```python
from build123d import *

# Parameters (mm, degrees)
F0_W     = 60
F0_H     = 40
F1_DEPTH = 10
F3_START = -20
F3_DEPTH = 20
F4_R     = 10
F5_DEPTH = 25


with BuildPart() as f1:
    # F0 (on Top) → F1 (new body)
    with BuildSketch(Plane.XY):
        with Locations((30, 20)):
            Rectangle(F0_W, F0_H)
    extrude(amount=F1_DEPTH)

    # F2 (on Front) → F3 (join)
    with BuildSketch(Plane.XZ.offset(F3_START)):
        with BuildLine():
            Line((50, 20), (40, 20))
            ThreePointArc((40, 20), (20, 40), (0, 20))
            Line((0, 20), (0, 10))
            Line((0, 10), (60, 10))
            ThreePointArc((60, 10), (57.0710678119, 17.0710678119), (50, 20))
        make_face()
    extrude(amount=-F3_DEPTH)

    # F4 (on face) → F5 (cut)
    with BuildSketch(Plane.XZ.offset(-20)):
        with Locations((20, 20)):
            Circle(F4_R)
    extrude(amount=-F5_DEPTH, mode=Mode.SUBTRACT)


solid = f1.part
```
Geometry check sheet. Reference: the model listing, model coordinates, mm. A direction names the side the tool comes from. Coordinates: 2 decimals unless noted, no trailing zeros. Order: outer loops, then holes, each group sorted by start corner. A loop starts at its lowest first (then second) coordinate and runs counter-clockwise, first axis right, second up. Notation, with made-up numbers: M 77,19.5 L 114,19.5 A18 cw 114,36.5 Z; hole C -18.75,7 d11. An arc over 180 degrees is marked long. One line per question, with ' | ' between items. Start each with the question number.
Item 1: Set-up check for faces 1 (the flat face through (30, 10, 10)), 2 (the cylindrical face through (57.15, 29.86, 16.99)): record each of +Z, -Z, +X, -X, +Y, -Y from which the full face is reachable in a straight line by a thin tool's end or side.
Item 2: Cross-section at B-B on z = 24.5. Enter the section's corners in (x, y), then the cut area to 3 significant figures.
Item 3: Cross-section at C-C on x = 41. Enter the section's corners in (y, z), then the cut area to 3 significant figures.
Item 4: Material ranges on L1, parallel to Z at x = 20, y = 32.25; L2, parallel to Y at x = 29, z = 32; L3, parallel to Z at x = 37.5, y = 12, recorded low to high. Write a range as [from, to].
Item 5: Gauge pin test, flat ends, axial feed: pin 1 (9 mm diameter, centred on x = 40.5, z = 23.5, fed in from -Y); pin 2 (22 mm diameter, centred on x = 36.5, y = 6, fed in from +Z); pin 3 (2 mm diameter, centred on y = 28.5, z = 28, fed in from +X) (3 decimals). Record the tip position at first contact, or that the pin passes through.
Item 6: Draft check along Z on faces 3 (the flat face through (30, 40, 16)), 4 (the cylindrical face through (29.54, 29.86, 23)), 5 (the flat face through (45, 30, 20)), 6 (the flat face through (30, 20, 0)). Enter one of: pulls with the +Z half, pulls with the -Z half, needs draft (parallel to the pull), parting line crosses it, or undercut.
Item 7: Cross-section at A-A on y = 23. Enter the section's corners in (x, z), then the cut area to 3 significant figures.
Item 8: Cross-section at D-D on x = 15. Enter the section's corners in (y, z), then the cut area to 3 significant figures.
Findings:
1) face 1: +Z, +X, -X, -Y | face 2: +Z, +X, +Y, -Y
2) outline: M 0.51,20 L 11.07,20 L 11.07,40 L 0.51,40 Z; M 28.93,20 L 39.49,20 L 39.49,40 L 28.93,40 Z | area: 422 mm²
3) outline: M 0,0 L 40,0 L 40,20 L 20,20 L 20,10 L 0,10 Z | area: 600 mm²
4) L1: z = [0, 10], [30, 40] | L2: y = [20, 40] | L3: z = [0, 10]
5) pin 1: stops at y = 20 | pin 2: stops at z = 10 | pin 3: stops at x = 38.735
6) face 3: needs draft | face 4: undercut | face 5: pulls with the +Z half | face 6: pulls with the -Z half
7) outline: M 0,0 L 60,0 L 60,10 A10 ccw 50,20 L 40,20 A20 ccw 0,20 Z; hole C 20,20 d20 | area: 1,490 mm²
8) outline: M 0,0 L 40,0 L 40,11.34 L 20,11.34 L 20,10 L 0,10 Z; M 20,28.66 L 40,28.66 L 40,39.36 L 20,39.36 Z | area: 641 mm²
